```python
from build123d import *

# Parameters (mm, degrees)
SKETCH1_R           = 1.5
BOSS_EXTRUDE1_DEPTH = 2
SKETCH2_W           = 18
SKETCH2_H           = 23.2
BOSS_EXTRUDE2_DEPTH = 2
CHAMFER1_SIZE       = 2


with BuildPart() as part:
    # Sketch1 → Boss-Extrude1 (new body)
    with BuildSketch(Plane.XY):
        with BuildLine():
            Line((-15, 11), (15, 11))
            ThreePointArc((15, 11), (26, 0), (15, -11))
            Line((15, -11), (-15, -11))
            ThreePointArc((-15, -11), (-26, 0), (-15, 11))
        make_face()
        with Locations((-15, 0)):
            Circle(SKETCH1_R, mode=Mode.SUBTRACT)
        with Locations((15, 0)):
            Circle(SKETCH1_R, mode=Mode.SUBTRACT)
        Circle(SKETCH1_R, mode=Mode.SUBTRACT)
    extrude(amount=BOSS_EXTRUDE1_DEPTH)

    # Sketch2 → Boss-Extrude2 (add)
    with BuildSketch(Plane(origin=(0, 11, 0), x_dir=(1, 0, 0), z_dir=(0, 1, 0))):
        with Locations((0, 9.6)):
            Rectangle(SKETCH2_W, SKETCH2_H)
    extrude(amount=BOSS_EXTRUDE2_DEPTH)

    # Chamfer1
    # the kernel refuses this chamfer: 2 mm, written as the material it takes off along each edge
    with BuildSketch(Plane(origin=(-9, 13, -26.343365976), x_dir=(-0.027495876610586487, -0.9996219169112968, 0), z_dir=(0, 0, 1)), Plane(origin=(9, 13, 7.143365976), x_dir=(0.027495876610586487, -0.9996219169112968, 0), z_dir=(0, 0, -1))) as chamfer1_piece_1:
        Polygon((CHAMFER1_SIZE * 0.999621916911, CHAMFER1_SIZE * 0.0274958766106), (-CHAMFER1_SIZE * 0.0274958766106, CHAMFER1_SIZE * 0.999621916911), (0, 0), align=None)
    extrude(amount=33.486731952, mode=Mode.SUBTRACT)


solid = part.part
```
The model under review builds one solid part; all positions refer to its coordinate system, in mm. A direction names the side the tool comes from. Round coordinates to 2 decimals unless told otherwise and drop trailing zeros. Loops run counter-clockwise (first coordinate to the right, second up) from the corner with the lowest first, then second, coordinate; pieces in that order, holes last.
1) Consider section A-A on x = 0. State the section outline as (y, z) points.
Values follow:
outline: (-11, 0) - (-1.5, 0) - (-1.5, 2) - (-11, 2) - close; (1.5, 0) - (11, 0) - (11, -21.2) - (13, -21.2) - (13, 2) - (1.5, 2) - close
2) Tool access review of faces 1 (the face through (26, 0, 1)), 2 (the face through (12, 11, 1)), 3 (the face through (-16.5, 0.07, 0.99)), 4 (the face through (0, 11, -11)), 5 (the face through (-12, 11, 1)): name each direction out of +Z, -Z, +X, -X, +Y, -Y from which nothing blocks a thin tool from reaching the whole face with its end or side.
Values follow:
face 1: +Z, -Z, +X
face 2: +Z, -Z, +X, +Y
face 3: +Z, -Z
face 4: -Z, +X, -X, -Y
face 5: +Z, -Z, -X, +Y
3) Wall thickness on line 1 along Y through (x, z) = (15, 1.25); line 2 along Y through (x, z) = (0, 0.6); line 3 along Z through (x, y) = (15.5, -8.5): over which ranges is each line inside the solid? List them lowest first.
Values follow:
line 1: y = -11 to -1.5, 1.5 to 11
line 2: y = -11 to -1.5, 1.5 to 13
line 3: z = 0 to 2
4) The part is to be moulded in two halves that separate along X. For faces 6 (the face through (-1.5, 0.07, 0.99)), 7 (the face through (8, 12, -9)), 8 (the face through (0, -2, 2)), say which applies: pulls with the +X half, pulls with the -X half, needs draft (parallel to the pull), parting line crosses it, or undercut.
Values follow:
face 6: undercut
face 7: pulls with the +X half
face 8: needs draft
5) Consider section D-D on x = 6. State the section outline as (y, z) points.
Values follow:
outline: (-11, 0) - (11, 0) - (11, -21.2) - (13, -21.2) - (13, 2) - (-11, 2) - close
6) Clearance check with flat-ended pins moving along their axes: P1, Ø2, axis at x = -6, z = -6, coming from the -Y side; P2, Ø4, axis at x = 0, y = 0, coming from the -Z side; P3, Ø1.6, axis at x = -13.5, z = 1, coming from the +Y side. State where each tip first meets the part, or that it passes through.
Values follow:
P1: stops at y = 11
P2: stops at z = 0
P3: stops at y = 11
7) Consider section B-B on y = 0. State the section outline as (x, z) points, then the cut area to 3 significant figures.
Values follow:
outline: (-26, 0) - (-16.5, 0) - (-16.5, 2) - (-26, 2) - close; (-13.5, 0) - (-1.5, 0) - (-1.5, 2) - (-13.5, 2) - close; (1.5, 0) - (13.5, 0) - (13.5, 2) - (1.5, 2) - close; (16.5, 0) - (26, 0) - (26, 2) - (16.5, 2) - close
area: 86.0 mm2
8) Consider section C-C on z = -5. State the section outline as (x, y) points, then the cut area to 3 significant figures.
Values follow:
outline: (-9, 11) - (9, 11) - (7, 13) - (-7, 13) - close
area: 32.0 mm2
